```python
from build123d import *

# Parameters (mm, degrees)
SKETCH1_W               = 33
SKETCH1_H               = 20
BOSS_EXTRUDE1_DEPTH     = 4
BOSS_EXTRUDE2_START     = -13
BOSS_EXTRUDE2_DEPTH     = 13
FILLET2_R               = 5.8
CUT_EXTRUDE1_DEPTH      = 59.600341412
CUT_EXTRUDE1_DEPTH_BACK = 59.600341412
SKETCH3_R               = 2.75
CUT_EXTRUDE2_DEPTH      = 24.26
FILLET3_R               = 40
SKETCH5_R               = 6
CUT_EXTRUDE3_DEPTH      = 5.96
SKETCH7_W               = 48
SKETCH7_H               = 16
CUT_EXTRUDE6_DEPTH      = 6
FILLET4_R               = 8
FILLET5_R               = 2
CUT_EXTRUDE7_DEPTH      = 57.550862204
CUT_EXTRUDE7_DEPTH_BACK = 57.550862204
SKETCH8_R               = 2.75


with BuildPart() as part:
    # Sketch1 → Boss-Extrude1 (new, symmetric)
    with BuildSketch(Plane.XY):
        with Locations((16.5, 0)):
            Rectangle(SKETCH1_W, SKETCH1_H)
    extrude(amount=BOSS_EXTRUDE1_DEPTH, both=True)

    # Sketch2 → Boss-Extrude2 (add)
    with BuildSketch(Plane(origin=(0, 10, 0), x_dir=(1, 0, 0), z_dir=(0, 1, 0)).offset(BOSS_EXTRUDE2_START)):
        with BuildLine():
            Line((33, 5), (33, -4))
            Line((33, -4), (47.358898944, -4))
            ThreePointArc((47.358898944, -4), (48.310885546, 13.473163206), (33, 5))
        make_face()
    extrude(amount=BOSS_EXTRUDE2_DEPTH)

    # Fillet2
    fillet2_edges = [part.edges().sort_by_distance(p)[0] for p in [
        (40.179449472, -3, 4),
    ]]
    fillet(fillet2_edges, radius=FILLET2_R)

    # Sketch3 → Cut-Extrude1 (cut, two sides: drawn at the far end of the back side and taken through both)
    with BuildSketch(Plane(origin=(0, 10, 0), x_dir=(1, 0, 0), z_dir=(0, 1, 0)).offset(-CUT_EXTRUDE1_DEPTH_BACK)):
        with Locations(Location((43, 5, 0), (0, 0, 180))):
            Circle(SKETCH3_R)
    extrude(amount=CUT_EXTRUDE1_DEPTH + CUT_EXTRUDE1_DEPTH_BACK, mode=Mode.SUBTRACT)

    # Sketch4 → Cut-Extrude2 (cut)
    with BuildSketch(Plane.XY.offset(4)):
        Polygon((33, 10), (53, 3.02413209), (53, 10), align=None)
    extrude(amount=-CUT_EXTRUDE2_DEPTH, mode=Mode.SUBTRACT)

    # Fillet3
    # the kernel refuses this fillet: 40 mm, written as the material it takes off along each edge
    with BuildSketch(Plane(origin=(33, 10, 20.939258542), x_dir=(0.9442130463798117, -0.32933527452454203, 0), z_dir=(0, 0, -1))) as fillet3_piece_1:
        with BuildLine():
            CenterArc((FILLET3_R * 0.169392585415, FILLET3_R), FILLET3_R, 250.771565663, 19.228434337)
            Line((-FILLET3_R * 0.159942689109, FILLET3_R * 0.0557869536202), (0, 0))
            Line((0, 0), (FILLET3_R * 0.169392585415, 0))
        make_face()
    extrude(amount=41.878517083, mode=Mode.SUBTRACT)

    # Sketch5 → Cut-Extrude3 (cut)
    with BuildSketch(Plane(origin=(0, 10, 0), x_dir=(1, 0, 0), z_dir=(0, 1, 0))):
        with Locations(Location((43, 5, 0), (0, 0, 180))):
            Circle(SKETCH5_R)
    extrude(amount=-CUT_EXTRUDE3_DEPTH, mode=Mode.SUBTRACT)

    # Mirror2: part across plane


with BuildPart() as part_1:
    add(part.part)
    add(part.part.mirror(Plane(origin=(0, 10, 4), x_dir=(0, 0, 1), z_dir=(1, 0, 0))))

    # Sketch7 → Cut-Extrude6 (cut)
    with BuildSketch(Plane(origin=(0, 0, -4), x_dir=(-1, 0, 0), z_dir=(0, 0, -1))):
        with Locations((0, -2)):
            Rectangle(SKETCH7_W, SKETCH7_H)
    extrude(amount=-CUT_EXTRUDE6_DEPTH, mode=Mode.SUBTRACT)

    # Fillet4
    fillet4_edges = [part_1.edges().sort_by_distance(p)[0] for p in [
        (-24, 6, -1),
        (24, 6, -1),
    ]]
    fillet(fillet4_edges, radius=FILLET4_R)

    # Fillet5
    fillet5_edges = [part_1.edges().sort_by_distance(p)[0] for p in [
        (-24, -6, 2),
        (0, 6, 2),
        (24, -6, 2),
        (21.656854249, 3.656854249, 2),
        (-21.656854249, 3.656854249, 2),
    ]]
    fillet(fillet5_edges, radius=FILLET5_R)

    # Sketch8 → Cut-Extrude7 (cut, two sides: drawn at the far end of the back side and taken through both)
    with BuildSketch(Plane(origin=(0, 0, 2), x_dir=(-1, 0, 0), z_dir=(0, 0, -1)).offset(-CUT_EXTRUDE7_DEPTH_BACK)):
        with Locations((-8, -2)):
            Circle(SKETCH8_R)
        with Locations((8, -2)):
            Circle(SKETCH8_R)
    extrude(amount=CUT_EXTRUDE7_DEPTH + CUT_EXTRUDE7_DEPTH_BACK, mode=Mode.SUBTRACT)


solid = part_1.part
```
For this review, take the finished solid that the model builds, in its own axes (mm). A direction names the side the tool comes from. Coordinates: 2 decimals unless noted, no trailing zeros. Loops run counter-clockwise (first coordinate to the right, second up) from the corner with the lowest first, then second, coordinate; pieces in that order, holes last.
1. Mouldability with a two-part tool opening along Y and no side actions: class faces 1 (the cylindrical face through (5.46, -3.05, 3.01)), 2 (the cylindrical face through (-34.28, 9.18, -3)), 3 (the cylindrical face through (-45.747, 0.471, -4.879)) as +Y half, -Y half, draft (parallel to the pull), parting line (faces both ways), or undercut.
2. Add section A-A, the plane x = -8. Give the boundary of the cut face in (y, z).
3. For faces 4 (the flat face through (42, 4.04, -8)), 5 (the flat face through (-43, -3, -8)), 6 (the flat face through (-49.126, 4.375, -3.256)), 7 (the cylindrical face through (0.22, 5.43, 1.4)), list the 3-axis set-ups (+Z, -Z, +X, -X, +Y, -Y) from which the entire face can be reached by the end or side of a thin tool; tool diameter is ignored.
4. Insertion check: P1, Ø6.5, axis at y = -1, z = -1.5, coming from the -X side; P2, Ø1, axis at y = 5.5, z = -8.5, coming from the +X side; P3, Ø3, axis at x = 11, z = -6, coming from the +Y side; P4, Ø4.5, axis at y = -7, z = -1.5, coming from the +X side. Each pin has a flat end and moves straight along its axis. Give the tip position at first contact, or say it passes through.
5. Add section C-C, the plane z = -8.75. Give the boundary of the cut face in (x, y).
6. Add section D-D, the plane x = -43. Give the boundary of the cut face in (y, z), then the cut area to 3 significant figures.
7. Add section B-B, the plane y = -7.75. Give the boundary of the cut face in (x, z), then the cut area to 3 significant figures.
8. For line 1 (Z direction, x = -43, y = 5.45); line 2 (X direction, y = 1.5, z = -5); line 3 (Y direction, x = -8, z = 2.85), list the stretches that pass through material, from the lowest coordinate up.
Result:
1. face 1: undercut
1. face 2: +Y half
1. face 3: draft
2. outline: (-10, 2) - (-4.75, 2) - (-4.75, 4) - (-10, 4) - close; (0.75, 2) - (4, 2) arc R2 cw to (6, 0) - (6, -4) - (10, -4) - (10, 4) - (0.75, 4) - close
3. face 4: +Y
3. face 5: +Z, -Z, -X, -Y
3. face 6: +Z, -Z, -X, +Y
3. face 7: -Z, -Y
4. P1: stops at x = -53
4. P2: stops at x = 38.53
4. P3: passes through
4. P4: stops at x = 33
5. outline: (-52.27, -3) - (-33.73, -3) - (-33.73, 9.29) arc R40 ccw to (-38.32, 8.13) - (-38.32, 4.04) - (-47.68, 4.04) - (-47.68, 4.88) - (-52.27, 3.28) - close; (33.73, -3) - (52.27, -3) - (52.27, 3.28) - (47.68, 4.88) - (47.68, 4.04) - (38.32, 4.04) - (38.32, 8.13) arc R40 ccw to (33.73, 9.29) - close
6. outline: (-3, -15) - (6.51, -15) - (6.51, -11) - (4.04, -11) - (4.04, -7.75) - (-3, -7.75) - close; (-3, -2.25) - (4.04, -2.25) - (4.04, 1) - (6.51, 1) - (6.51, 4) - (2.8, 4) arc R5.8 ccw to (-3, -1.8) - close
6. area: 105 mm2
7. outline: (-33, -4) - (-24, -4) - (-24, 0) arc R2 cw to (-22, 2) - (22, 2) arc R2 cw to (24, 0) - (24, -4) - (33, -4) - (33, 4) - (-33, 4) - close
7. area: 242 mm2
8. line 1: z = -15 to -11, 1 to 4
8. line 2: x = -53 to -45.75, -40.25 to -33, 33 to 40.25, 45.75 to 53
8. line 3: y = -10 to -4.75, 0.75 to 10
